Input: part model. Units: mm. Frame: model coordinates. Give positions to 0.01 mm unless a question says otherwise; leave off trailing zeros. Loops run counter-clockwise (first coordinate to the right, second up) from the corner with the lowest first, then second, coordinate; pieces in that order, holes last.
from build123d import *

# Parameters (mm, degrees)
F2_R = 2.99999
F3_R = 5


# Not quite as in the source:
# - a fillet or chamfer is up to 0.001 mm smaller than in the source, because OpenCascade refuses the exact size


with BuildPart() as f1:
    # F0 (on Front) → F1 (revolve)
    with BuildSketch(Plane.XZ):
        Polygon((-91.4914906025, 49.9999961555), (-94.4914906025, 49.9999961555), (-94.4914906025, -41.0000038445), (-47.6173348725, -41.0000038445), (-47.6173348725, -35.0000038445), (-91.4914906025, -35.0000038445), align=None)
    revolve(axis=Axis((-47.6173348725, 0, -38.0000038445), (0, 0, 1)))

    # F2 (radius 3 in the source; OpenCascade refuses exactly that, so slightly less here)
    f2_edges = [f1.edges().sort_by_distance(p)[0] for p in [
        (-0.743179, 0, 49.999996),
    ]]
    fillet(f2_edges, radius=F2_R)

    # F3
    f3_edges = [f1.edges().sort_by_distance(p)[0] for p in [
        (-0.743179, 0, -41.000004),
    ]]
    fillet(f3_edges, radius=F3_R)


solid = f1.part
(1) Cut plane B-B (z = -24). Return the cut outline in (x, y), and give its area (3 significant figures).
Values follow:
outline: circle Ø93.75 at (-47.62, 0); hole circle Ø87.75 at (-47.62, 0)
area: 855 mm2
(2) Pin query (flat end, axial travel): pin 1 Ø1 at (x, z) = (-34.5, 23.5) entering from -Y; pin 2 Ø8 at (x, z) = (-17, -12.5) entering from +Y; pin 3 Ø1.5 at (x, y) = (-15.5, 2.5) entering from +Z; pin 4 Ø3 at (y, z) = (-1.5, -17) entering from -X. Return the tip coordinate at first contact, or that it passes through.
Values follow:
pin 1: stops at y = -45.14
pin 2: stops at y = 38.58
pin 3: stops at z = -35
pin 4: stops at x = -94.49
(3) Mould query, pull axis X, two halves, no side actions, for faces 1 (the cylindrical face through (-37.46, 45.76, 4.92)), 2 (the flat face through (-47, -1, -41)), 3 (the flat face through (-48, -1, -35)). Classes: +X half, -X half, draft (parallel to the pull), parting line (faces both ways), or undercut.
Values follow:
face 1: parting line
face 2: draft
face 3: undercut
(4) Ray query, probe 1 along X at (y, z) = (0, 20); probe 2 along Z at (x, y) = (-40.5, 35.5); probe 3 along X at (y, z) = (29, 31.5). Return the intervals inside material, ascending.
Values follow:
probe 1: x = -94.49 to -91.49, -3.74 to -0.74
probe 2: z = -41 to -35
probe 3: x = -84.44 to -80.54, -14.69 to -10.79
